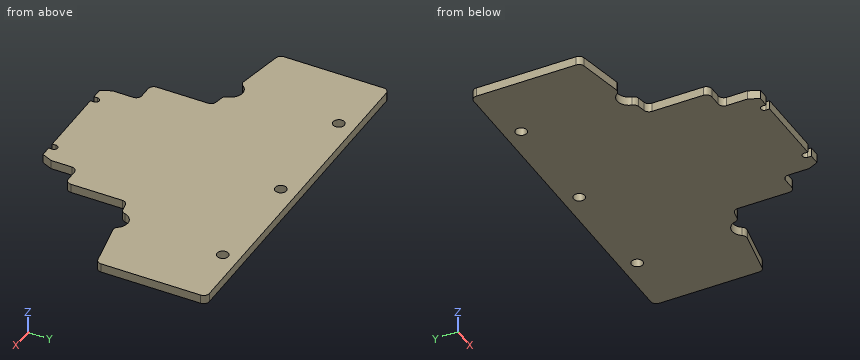
```python
from build123d import *

# Parameters (mm, degrees)
SKETCH1_W           = 80
SKETCH1_H           = 60
BOSS_EXTRUDE1_DEPTH = 1.6
SKETCH2_OUTSIDE_W   = 102.002
SKETCH2_OUTSIDE_H   = 82.002
CUT_EXTRUDE1_DEPTH  = 1.6
FILLET1_R           = 1
SKETCH3_R           = 1
CUT_EXTRUDE2_DEPTH  = 10


with BuildPart() as part:
    # Sketch1 → Boss-Extrude1 (new body)
    with BuildSketch(Plane.XY):
        with Locations((40, 30)):
            Rectangle(SKETCH1_W, SKETCH1_H)
    extrude(amount=BOSS_EXTRUDE1_DEPTH)

    # Sketch2 outside → Cut-Extrude1 (cut)
    with BuildSketch(Plane.XY.offset(1.6)):
        with Locations((40, 30)):
            Rectangle(SKETCH2_OUTSIDE_W, SKETCH2_OUTSIDE_H)
        with BuildLine():
            Line((8.830524125, 49.648617791), (70.632878184, 49.648617791))
            Line((70.632878184, 49.648617791), (70.632878184, 30.112540158))
            Line((70.632878184, 30.112540158), (61.123106489, 28.255784683))
            ThreePointArc((61.123106489, 28.255784683), (58.77201565, 29.627241667), (57.109476194, 27.472134952))
            Line((57.109476194, 27.472134952), (54.224418996, 26.908835862))
            Line((54.224418996, 26.908835862), (54.224418996, 15.955223451))
            Line((54.224418996, 15.955223451), (50.114060899, 15.955223451))
            Line((50.114060899, 15.955223451), (50.114060899, 11.256501231))
            Line((50.114060899, 11.256501231), (49.289397665, 9.401008955))
            Line((49.289397665, 9.401008955), (47.389901446, 9.401008955))
            Line((47.389901446, 9.401008955), (47.389901446, 10.047799846))
            ThreePointArc((47.389901446, 10.047799846), (46.783221619, 10.654479673), (46.176541793, 10.047799846))
            Line((46.176541793, 10.047799846), (46.176541793, 9.401008955))
            Line((46.176541793, 9.401008955), (33.286860516, 9.401008955))
            Line((33.286860516, 9.401008955), (33.286860516, 10.047799846))
            ThreePointArc((33.286860516, 10.047799846), (32.68018069, 10.654479673), (32.073500863, 10.047799846))
            Line((32.073500863, 10.047799846), (32.073500863, 9.401008955))
            Line((32.073500863, 9.401008955), (30.174004644, 9.401008955))
            Line((30.174004644, 9.401008955), (29.34934141, 11.256501231))
            Line((29.34934141, 11.256501231), (29.34934141, 15.955223451))
            Line((29.34934141, 15.955223451), (25.238983313, 15.955223451))
            Line((25.238983313, 15.955223451), (25.238983313, 26.908835862))
            Line((25.238983313, 26.908835862), (22.353926115, 27.472134952))
            ThreePointArc((22.353926115, 27.472134952), (20.691386659, 29.627241667), (18.34029582, 28.255784683))
            Line((18.34029582, 28.255784683), (8.830524125, 30.112540158))
            Line((8.830524125, 30.112540158), (8.830524125, 49.648617791))
        make_face(mode=Mode.SUBTRACT)
    extrude(amount=-CUT_EXTRUDE1_DEPTH, mode=Mode.SUBTRACT)

    # Fillet1
    fillet1_edges = [part.edges().sort_by_distance(p)[0] for p in [
        (8.830524125, 49.648617791, 0.8),
        (70.632878184, 49.648617791, 0.8),
        (70.632878184, 30.112540158, 0.8),
        (61.123106489, 28.255784683, 0.8),
        (57.109476194, 27.472134952, 0.8),
        (54.224418996, 26.908835862, 0.8),
        (54.224418996, 15.955223451, 0.8),
        (50.114060899, 15.955223451, 0.8),
        (29.34934141, 15.955223451, 0.8),
        (25.238983313, 15.955223451, 0.8),
        (25.238983313, 26.908835862, 0.8),
        (22.353926115, 27.472134952, 0.8),
        (18.34029582, 28.255784683, 0.8),
        (8.830524125, 30.112540158, 0.8),
    ]]
    fillet(fillet1_edges, radius=FILLET1_R)

    # Sketch3 → Cut-Extrude2 (cut)
    with BuildSketch(Plane.XY.offset(1.6)):
        with Locations((20.4, 46.768617791)):
            Circle(SKETCH3_R)
        with Locations((40, 46.768617791)):
            Circle(SKETCH3_R)
        with Locations((59.6, 46.768617791)):
            Circle(SKETCH3_R)
    extrude(amount=-CUT_EXTRUDE2_DEPTH, mode=Mode.SUBTRACT)


solid = part.part
```
The model under review builds one solid part; all positions refer to its coordinate system, in mm. Round coordinates to 2 decimals unless told otherwise and drop trailing zeros. Loops run counter-clockwise (first coordinate to the right, second up) from the corner with the lowest first, then second, coordinate; pieces in that order, holes last. Notation, with made-up numbers: (-10.5, -16) -> (23.5, -16) arc R27 cw to (23.5, 8) -> close; hole circle Ø6 at (-7.5, -10). An arc over 180 degrees is marked (long way). Answer in a Markdown table with one row per item.
1) Wall thickness on line 1 along Y through (x, z) = (20.4, 0.5); line 2 along Y through (x, z) = (40, 1.1); line 3 along X through (y, z) = (46.5, 0.2): over which ranges is each line inside the solid? List them lowest first.
Taken from the geometry:
| item | result |
|---|---|
| line 1 | y = 29.66 to 45.77, 47.77 to 49.65 |
| line 2 | y = 9.4 to 45.77, 47.77 to 49.65 |
| line 3 | x = 8.83 to 19.44, 21.36 to 39.04, 40.96 to 58.64, 60.56 to 70.63 |
2) Consider section A-A, the plane x = 40. Write out the cut boundary in (y, z), plus the area to 3 significant figures.
Taken from the geometry:
| item | result |
|---|---|
| outline | (9.4, 0) -> (45.77, 0) -> (45.77, 1.6) -> (9.4, 1.6) -> close; (47.77, 0) -> (49.65, 0) -> (49.65, 1.6) -> (47.77, 1.6) -> close |
| area | 61.2 mm² |
3) Consider section B-B, the plane y = 25. Write out the cut boundary in (x, z), plus the area to 3 significant figures.
Taken from the geometry:
| item | result |
|---|---|
| outline | (25.24, 0) -> (54.22, 0) -> (54.22, 1.6) -> (25.24, 1.6) -> close |
| area | 46.4 mm² |
4) Consider section C-C, the plane x = 20.4. Write out the cut boundary in (y, z), plus the area to 3 significant figures.
Taken from the geometry:
| item | result |
|---|---|
| outline | (29.66, 0) -> (45.77, 0) -> (45.77, 1.6) -> (29.66, 1.6) -> close; (47.77, 0) -> (49.65, 0) -> (49.65, 1.6) -> (47.77, 1.6) -> close |
| area | 28.8 mm² |
5) Consider section D-D, the plane z = 1.3. Count the separate pieces of the cut face and the enclosed holes in it, plus the area to 3 significant figures.
Taken from the geometry:
| item | result |
|---|---|
| separate pieces | 1 |
| enclosed holes | 3 |
| area | 1,780 mm² |
6) For pin 1 Ø0.8 at (y, z) = (13, 1) entering from +X; pin 2 Ø0.8 at (y, z) = (14, 1) entering from -X; pin 3 Ø0.7 at (y, z) = (9.5, 1) entering from +X, all flat-tipped, find the tip position at first contact; note any pin that passes through.
Taken from the geometry:
| item | result |
|---|---|
| pin 1 | stops at x = 50.11 |
| pin 2 | stops at x = 29.35 |
| pin 3 | stops at x = 49.49 |
